```python
from build123d import *

# Parameters (mm, degrees)
SKETCH1_W           = 254
SKETCH1_H           = 50.8
SKETCH1_R           = 15.24
BOSS_EXTRUDE1_DEPTH = 4.7498


with BuildPart() as part:
    # Sketch1 → Boss-Extrude1 (new body)
    # profile 1 of 3: a face of its own
    with BuildSketch(Plane(origin=(0, 0, 0), x_dir=(1, 0, 0), z_dir=(0, 1, 0))):
        with Locations((127, -25.4)):
            Rectangle(SKETCH1_W, SKETCH1_H)
        with Locations((127, -25.4)):
            Circle(SKETCH1_R, mode=Mode.SUBTRACT)
    # profile 2 of 3: a face of its own
    with BuildSketch(Plane(origin=(0, 0, 0), x_dir=(1, 0, 0), z_dir=(0, 1, 0))):
        with BuildLine():
            ThreePointArc((137.776307345, -14.623692655), (127, -10.16), (116.223692655, -14.623692655))
            Line((116.223692655, -14.623692655), (137.776307345, -14.623692655))
        make_face()
    # profile 3 of 3: a face of its own
    with BuildSketch(Plane(origin=(0, 0, 0), x_dir=(1, 0, 0), z_dir=(0, 1, 0))):
        with BuildLine():
            ThreePointArc((116.223692655, -36.176307345), (127, -40.64), (137.776307345, -36.176307345))
            Line((137.776307345, -36.176307345), (116.223692655, -36.176307345))
        make_face()
    extrude(amount=BOSS_EXTRUDE1_DEPTH)


solid = part.part
```
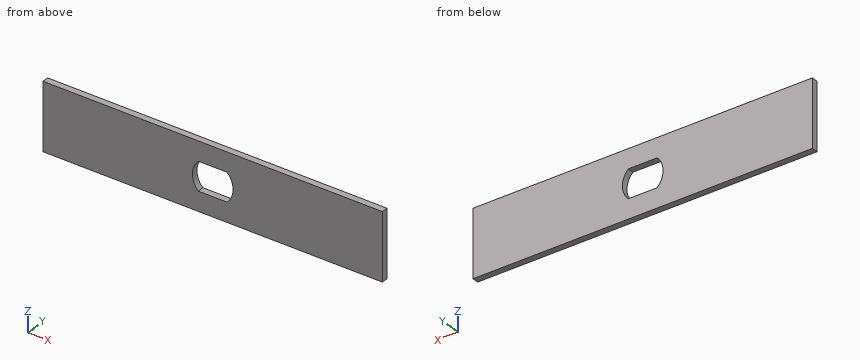
The listing builds one solid part. Answer for the finished solid, in the listing's coordinates (mm). Coordinates: 2 decimals unless noted, no trailing zeros. Write each loop counter-clockwise with the first axis right and the second up, starting at its lowest first coordinate (ties: lowest second). Pieces come first, ordered by that corner, then holes. Notation, with made-up numbers: (77.5, 11) - (101.5, 11) arc R12 cw to (101.5, 19) - close; hole circle Ø3 at (36.25, 14.25). An arc over 180 degrees is marked (long way). One line per item, written item: value.
1) Find section B-B (y = 3.1). Give the vertices of the cut face in (x, z).
Geometry check:
outline: (0, 0) - (254, 0) - (254, 50.8) - (0, 50.8) - close; hole (116.22, 14.62) - (137.78, 14.62) arc R15.24 ccw to (137.78, 36.18) - (116.22, 36.18) arc R15.24 ccw to start
2) This flat-tipped pin is pushed along its axis until it touches: pin 1 Ø2 at (x, z) = (185, 39) entering from -Y. Where does it stop, or does it pass through?
Geometry check:
pin 1: stops at y = 0
3) Find section A-A (x = 120). Give the vertices of the cut face in (y, z).
Geometry check:
outline: (0, 0) - (4.75, 0) - (4.75, 14.62) - (0, 14.62) - close; (0, 36.18) - (4.75, 36.18) - (4.75, 50.8) - (0, 50.8) - close
4) Consider line 1 along Z through (x, y) = (130, 1.7); line 2 along X through (y, z) = (4.4, 25.5); line 3 along X through (y, z) = (1.6, 27.5). Determine where each line is inside the solid, lowest interval first. Write a range as from..to.
Geometry check:
line 1: z = 0..14.62, 36.18..50.8
line 2: x = 0..111.76, 142.24..254
line 3: x = 0..111.91, 142.09..254
5) Find section C-C (z = 20.5). Give the vertices of the cut face in (x, y).
Geometry check:
outline: (0, 0) - (112.57, 0) - (112.57, 4.75) - (0, 4.75) - close; (141.43, 0) - (254, 0) - (254, 4.75) - (141.43, 4.75) - close
